Model file for the job. Use its own axes, mm. Round coordinates to 2 decimals unless told otherwise and drop trailing zeros. Loops run counter-clockwise (first coordinate to the right, second up) from the corner with the lowest first, then second, coordinate; pieces in that order, holes last. Notation, with made-up numbers: M 24.25,65 L 35.25,65 A21 cw 35.25,79 Z; hole C -22,-34 d1. An arc over 180 degrees is marked long. Answer in a Markdown table with one row per item.
from build123d import *

# Parameters (mm, degrees)
SKETCH_1_R               = 60
SKETCH_1_R_2             = 30
EXTRUDE_1_DEPTH          = 5.5
CUT_EXTRUDE_1_DEPTH      = 86.030876745
CUT_EXTRUDE_1_DEPTH_BACK = 86.030876745
SKETCH_2_R               = 2.5
CUT_EXTRUDE_3_DEPTH      = 86.030876745
CUT_EXTRUDE_3_DEPTH_BACK = 86.030876745
SKETCH_3_R               = 1.6


with BuildPart() as part:
    # ｽｹｯﾁ1 → ﾎﾞｽ - 押し出し1 (new body)
    with BuildSketch(Plane.XY):
        Circle(SKETCH_1_R)
        Circle(SKETCH_1_R_2, mode=Mode.SUBTRACT)
    extrude(amount=EXTRUDE_1_DEPTH)

    # ｽｹｯﾁ2 → ｶｯﾄ - 押し出し1 (cut, two sides: drawn at the far end of the back side and taken through both)
    with BuildSketch(Plane.XY.offset(5.5).offset(-CUT_EXTRUDE_1_DEPTH_BACK)):
        with Locations((0, -50)):
            Circle(SKETCH_2_R)
        with Locations((-50, 0)):
            Circle(SKETCH_2_R)
        with Locations((50, 0)):
            Circle(SKETCH_2_R)
        with Locations((0, 50)):
            Circle(SKETCH_2_R)
    extrude(amount=CUT_EXTRUDE_1_DEPTH + CUT_EXTRUDE_1_DEPTH_BACK, mode=Mode.SUBTRACT)

    # ｽｹｯﾁ3 → ｶｯﾄ - 押し出し3 (cut, two sides: drawn at the far end of the back side and taken through both)
    with BuildSketch(Plane.XY.offset(5.5).offset(-CUT_EXTRUDE_3_DEPTH_BACK)):
        with Locations((30.245839942, 25)):
            Circle(SKETCH_3_R)
        with Locations((-30.245839942, 25)):
            Circle(SKETCH_3_R)
        with Locations((-30.245839942, -25)):
            Circle(SKETCH_3_R)
        with Locations((30.245839942, -25)):
            Circle(SKETCH_3_R)
    extrude(amount=CUT_EXTRUDE_3_DEPTH + CUT_EXTRUDE_3_DEPTH_BACK, mode=Mode.SUBTRACT)


solid = part.part
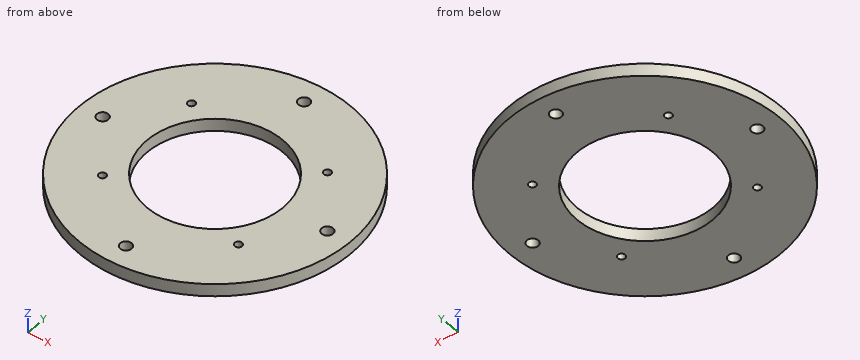
1. Wall check: probe 1 along Y at (x, z) = (0, 2.5); probe 2 along X at (y, z) = (-25, 2.1); probe 3 along Y at (x, z) = (31.5, 3.25). Give the ranges that are in metal, low to high.
Verdict:
| item | result |
|---|---|
| probe 1 | y = -60 to -52.5, -47.5 to -30, 30 to 47.5, 52.5 to 60 |
| probe 2 | x = -54.54 to -31.85, -28.65 to -16.58, 16.58 to 28.65, 31.85 to 54.54 |
| probe 3 | y = -51.07 to -25.99, -24.01 to 24.01, 25.99 to 51.07 |
2. Saw through at A-A (z = 1.65). State how many separate pieces and enclosed holes the cut face has, and give its area (3 significant figures).
Verdict:
| item | result |
|---|---|
| separate pieces | 1 |
| enclosed holes | 9 |
| area | 8,370 mm² |
3. Saw through at D-D (x = 16). Write the cut outline in (y, z), and give its area (3 significant figures).
Verdict:
| item | result |
|---|---|
| outline | M -57.83,0 L -25.38,0 L -25.38,5.5 L -57.83,5.5 Z; M 25.38,0 L 57.83,0 L 57.83,5.5 L 25.38,5.5 Z |
| area | 357 mm² |
4. Saw through at C-C (y = 50). Write the cut outline in (x, z).
Verdict:
| item | result |
|---|---|
| outline | M -33.17,0 L -2.5,0 L -2.5,5.5 L -33.17,5.5 Z; M 2.5,0 L 33.17,0 L 33.17,5.5 L 2.5,5.5 Z |
5. Saw through at B-B (y = 0). Write the cut outline in (x, z), and give its area (3 significant figures).
Verdict:
| item | result |
|---|---|
| outline | M -60,0 L -52.5,0 L -52.5,5.5 L -60,5.5 Z; M -47.5,0 L -30,0 L -30,5.5 L -47.5,5.5 Z; M 30,0 L 47.5,0 L 47.5,5.5 L 30,5.5 Z; M 52.5,0 L 60,0 L 60,5.5 L 52.5,5.5 Z |
| area | 275 mm² |
6. Pin check, flat tip, straight feed: pin 1 (3 mm diameter, centred on y = -8.5, z = 3, fed in from -X). Stop position of the tip, or through.
Verdict:
| item | result |
|---|---|
| pin 1 | stops at x = -59.59 |
